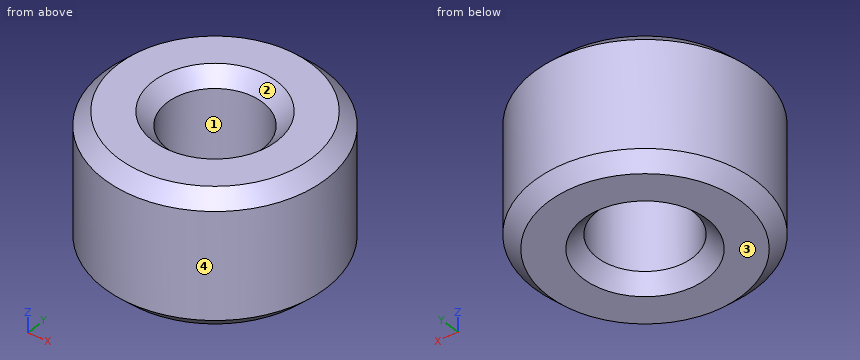
```python
from build123d import *

# Parameters (mm, degrees)
CROQUIS1_R              = 3.95
CROQUIS1_R_2            = 1.7
SALIENTE_EXTRUIR1_DEPTH = 4.8
CHAFL_N1_SIZE           = 0.5


with BuildPart() as part:
    # Croquis1 → Saliente-Extruir1 (new body)
    with BuildSketch(Plane.XY):
        with Locations((-7.600000242, 9.362000442)):
            Circle(CROQUIS1_R)
        with Locations((-7.600000242, 9.362000442)):
            Circle(CROQUIS1_R_2, mode=Mode.SUBTRACT)
    extrude(amount=SALIENTE_EXTRUIR1_DEPTH)

    # Chaflán1
    chafl_n1_edges = [part.edges().sort_by_distance(p)[0] for p in [
        (-11.550000242, 9.362000442, 0),
        (-11.550000242, 9.362000442, 4.8),
        (-9.300000242, 9.362000442, 0),
        (-9.300000242, 9.362000442, 4.8),
    ]]
    chamfer(chafl_n1_edges, length=CHAFL_N1_SIZE)


solid = part.part
```
Verification items for the finished model (mm, model axes). Face numbers are marked on the shaded views. Round coordinates to 2 decimals unless told otherwise and drop trailing zeros. Write each loop counter-clockwise with the first axis right and the second up, starting at its lowest first coordinate (ties: lowest second). Pieces come first, ordered by that corner, then holes. Notation, with made-up numbers: (-32, 42) - (14, 42) arc R17 cw to (14, 66) - close; hole circle Ø2 at (33.25, 87). An arc over 180 degrees is marked (long way). Answer as a JSON object with one key per item and string values. Group by question number.
Q1. Section check B-B, the plane z = 2.95. Enter the section's corners in (x, y), plus the area to 3 significant figures.
Q2. Mould release check, pull along X, two halves, no side actions. Record for the marked faces 1, 2, 3 and 4: released by +X, released by -X, zero draft, split by the parting line, or undercut.
Q3. Go/stop test with flat-tipped pins: pin 1 Ø1 at (x, y) = (-9, 9.5) entering from +Z; pin 2 Ø1.5 at (x, y) = (-7.5, 10.5) entering from -Z; pin 3 Ø3 at (x, y) = (-7.6, 9.362) entering from +Z. Record where each tip stops, or that it passes through.
Q4. Section check A-A, the plane x = -7.6. Enter the section's corners in (y, z), plus the area to 3 significant figures.
Q5. Thickness scan on line 1 (Y direction, x = -7.6, z = 3); line 2 (Y direction, x = -9, z = 0.6); line 3 (X direction, y = 9.25, z = 2.05). Record the ranges inside material, lowest first.
Found:
{
 "1": {"outline": "circle Ø7.9 at (-7.6, 9.36); hole circle Ø3.4 at (-7.6, 9.36)", "area": "39.9 mm^2"},
 "2": {"face 1": "undercut", "face 2": "undercut", "face 3": "zero draft", "face 4": "split by the parting line"},
 "3": {"pin 1": "stops at z = 4.51", "pin 2": "stops at z = 0.31", "pin 3": "passes through"},
 "4": {"outline": "(5.41, 0.5) - (5.91, 0) - (7.16, 0) - (7.66, 0.5) - (7.66, 4.3) - (7.16, 4.8) - (5.91, 4.8) - (5.41, 4.3) - close; (11.06, 0.5) - (11.56, 0) - (12.81, 0) - (13.31, 0.5) - (13.31, 4.3) - (12.81, 4.8) - (11.56, 4.8) - (11.06, 4.3) - close", "area": "20.6 mm^2"},
 "5": {"line 1": "y = 5.41 to 7.66, 11.06 to 13.31", "line 2": "y = 5.67 to 8.4, 10.33 to 13.06", "line 3": "x = -11.55 to -9.3, -5.9 to -3.65"}
}
